```python
from build123d import *

# Parameters (mm, degrees)
SKETCH008_W     = 36.83
SKETCH008_H     = 68.58
PAD006_DEPTH    = 8.89
SKETCH009_W     = 31.75
SKETCH009_H     = 62.23
POCKET001_DEPTH = 6.35
SKETCH010_R     = 5.715
SKETCH010_W     = 6.35
SKETCH010_H     = 2.54
SKETCH010_W_2   = 5.08
SKETCH010_W_3   = 2.54
SKETCH010_H_2   = 6.35
SKETCH010_H_3   = 3.81
PAD007_DEPTH    = 6.35
POCKET002_DEPTH = 1.5875
SKETCH012_W     = 36.83
SKETCH012_H     = 68.58
SKETCH012_W_2   = 31.75
SKETCH012_H_2   = 62.23
SKETCH012_R     = 5.715
PAD008_DEPTH    = 3.81
SKETCH013_R     = 5.08
POCKET003_DEPTH = 5.08
SKETCH014_R     = 1.651
POCKET004_DEPTH = 12.701
SKETCH015_R     = 3.175
POCKET005_DEPTH = 10.16
SKETCH016_R     = 3.175
POCKET006_DEPTH = 4.7625
SKETCH017_W     = 5.715
SKETCH017_H     = 1.143
PAD009_DEPTH    = 1.27
POCKET007_DEPTH = 10.16
SKETCH019_W     = 29.21
SKETCH019_H     = 1.143
SKETCH019_W_2   = 5.08
PAD010_DEPTH    = 1.27
FILLET004_R     = 1.27
FILLET005_R     = 0.762


with BuildPart() as part:
    # Sketch008 → Pad006 (new body)
    with BuildSketch(Plane.XY):
        with Locations((15.875, 31.75)):
            Rectangle(SKETCH008_W, SKETCH008_H)
    extrude(amount=-PAD006_DEPTH)

    # Sketch009 (on Face5 of Pad006) → Pocket001 (cut)
    with BuildSketch(Plane.XY):
        with Locations((15.875, 31.115)):
            Rectangle(SKETCH009_W, SKETCH009_H)
    extrude(amount=-POCKET001_DEPTH, mode=Mode.SUBTRACT)

    # Sketch010 (on Face11 of Pocket001) → Pad007 (join)
    with BuildSketch(Plane.XY.offset(-6.35)):
        with Locations((7.62, 22.225)):
            Circle(SKETCH010_R)
        with Locations((7.62, 50.8)):
            Circle(SKETCH010_R)
        with Locations((24.13, 50.8)):
            Circle(SKETCH010_R)
        with Locations((3.175, 33.02)):
            Rectangle(SKETCH010_W, SKETCH010_H)
        with Locations((29.21, 33.02)):
            Rectangle(SKETCH010_W_2, SKETCH010_H)
        with Locations((3.175, 9.525)):
            Rectangle(SKETCH010_W, SKETCH010_H)
        with Locations((29.21, 9.525)):
            Rectangle(SKETCH010_W_2, SKETCH010_H)
        with Locations((15.875, 37.465)):
            Rectangle(SKETCH010_W_3, SKETCH010_H_2)
        with Locations((13.97, 1.905)):
            Rectangle(SKETCH010_W_3, SKETCH010_H_3)
    extrude(amount=PAD007_DEPTH)

    # Sketch011 (on Face4 of Pad007) → Pocket002 (cut)
    with BuildSketch(Plane.XY):
        with BuildLine():
            Line((2.286, 0), (31.369, 0))
            Line((31.369, 0), (31.369, 38.608))
            Line((31.369, 38.608), (2.286, 38.608))
            Line((2.286, 38.608), (2.286, 25.670424))
            ThreePointArc((2.286, 25.670424), (1.27, 22.225), (2.286, 18.779576))
            Line((2.286, 0), (2.286, 18.779576))
        make_face()
    extrude(amount=-POCKET002_DEPTH, mode=Mode.SUBTRACT)

    # Sketch012 (on Face4 of Pocket002) → Pad008 (join)
    with BuildSketch(Plane.XY):
        with Locations((15.875, 31.75)):
            Rectangle(SKETCH012_W, SKETCH012_H)
        with Locations((15.875, 31.115)):
            Rectangle(SKETCH012_W_2, SKETCH012_H_2, mode=Mode.SUBTRACT)
        with Locations((7.62, 50.8)):
            Circle(SKETCH012_R)
        with Locations((24.13, 50.8)):
            Circle(SKETCH012_R)
    extrude(amount=PAD008_DEPTH)

    # Sketch013 (on Face4 of Pad008) → Pocket003 (cut)
    with BuildSketch(Plane.XZ.offset(2.54)):
        with Locations((23.495, 3.81)):
            Circle(SKETCH013_R)
        with BuildLine():
            Line((2.54, 3.81), (3.556, 2.54))
            Line((3.556, 2.54), (4.826, 2.54))
            ThreePointArc((4.826, 2.54), (7.62, -0.254), (10.414, 2.54))
            Line((10.414, 2.54), (11.684, 2.54))
            Line((11.684, 2.54), (12.7, 3.81))
            Line((12.7, 3.81), (2.54, 3.81))
        make_face()
    extrude(amount=-POCKET003_DEPTH, mode=Mode.SUBTRACT)

    # Sketch014 (on Face11 of Pocket003) → Pocket004 (cut, through all)
    with BuildSketch(Plane.XY.offset(3.81)):
        with Locations((7.62, 50.8)):
            Circle(SKETCH014_R)
        with Locations((24.13, 50.8)):
            Circle(SKETCH014_R)
        with Locations((7.62, 22.225)):
            Circle(SKETCH014_R)
    extrude(amount=-POCKET004_DEPTH, mode=Mode.SUBTRACT)

    # Sketch015 (on Face8 of Pocket004) → Pocket005 (cut)
    with BuildSketch(Plane(origin=(0, 0, -8.89), x_dir=(1, 0, 0), z_dir=(0, 0, -1))):
        with Locations((7.62, -50.8)):
            Circle(SKETCH015_R)
        with Locations((24.13, -50.8)):
            Circle(SKETCH015_R)
    extrude(amount=-POCKET005_DEPTH, mode=Mode.SUBTRACT)

    # Sketch016 (on Face8 of Pocket005) → Pocket006 (cut)
    with BuildSketch(Plane(origin=(0, 0, -8.89), x_dir=(1, 0, 0), z_dir=(0, 0, -1))):
        with Locations((7.62, -22.225)):
            Circle(SKETCH016_R)
    extrude(amount=-POCKET006_DEPTH, mode=Mode.SUBTRACT)

    # Sketch017 (on Face11 of Pocket006) → Pad009 (join)
    with BuildSketch(Plane.XY.offset(3.81)):
        Polygon((0, 62.23), (-1.143, 62.23), (-1.143, -1.143), (2.54, -1.143), (2.54, 0), (0, 0), align=None)
        Polygon((31.75, 62.23), (31.75, 0), (28.575, 0), (28.575, -1.143), (32.893, -1.143), (32.893, 62.23), align=None)
        with Locations((15.5575, -0.5715)):
            Rectangle(SKETCH017_W, SKETCH017_H)
    extrude(amount=PAD009_DEPTH)

    # Sketch018 (on Face11 of Pad009) → Pocket007 (cut)
    with BuildSketch(Plane.XY.offset(3.81)):
        Polygon((1.27, 66.04), (1.27, 64.897), (0, 64.897), (0, 63.373), (1.27, 63.373), (1.27, 62.23), (30.48, 62.23), (30.48, 63.373), (31.75, 63.373), (31.75, 64.897), (30.48, 64.897), (30.48, 66.04), align=None)
    extrude(amount=-POCKET007_DEPTH, mode=Mode.SUBTRACT)

    # Sketch019 (on Face63 of Pocket007) → Pad010 (join)
    with BuildSketch(Plane.XY.offset(-6.35)):
        with Locations((15.875, 65.4685)):
            Rectangle(SKETCH019_W, SKETCH019_H)
        with Locations((3.81, 62.8015)):
            Rectangle(SKETCH019_W_2, SKETCH019_H)
        with Locations((27.94, 62.8015)):
            Rectangle(SKETCH019_W_2, SKETCH019_H)
    extrude(amount=PAD010_DEPTH)

    # Fillet004
    fillet004_edges = [part.edges().sort_by_distance(p)[0] for p in [
        (-2.54, -2.54, 1.905),
        (-2.54, -2.54, -4.445),
        (34.29, -2.54, -4.445),
        (34.29, -2.54, 1.905),
        (34.29, 66.04, 1.905),
        (34.29, 66.04, -4.445),
        (15.875, -2.54, -8.89),
        (34.29, 31.75, -8.89),
        (-2.54, 31.75, -8.89),
        (15.875, 66.04, -8.89),
        (-2.54, 66.04, 1.905),
        (-2.54, 66.04, -4.445),
    ]]
    fillet(fillet004_edges, radius=FILLET004_R)

    # Fillet005
    fillet005_edges = [part.edges().sort_by_distance(p)[0] for p in [
        (4.445, 22.225, -8.89),
        (20.955, 50.8, -8.89),
        (4.445, 50.8, -8.89),
    ]]
    fillet(fillet005_edges, radius=FILLET005_R)


solid = part.part
```
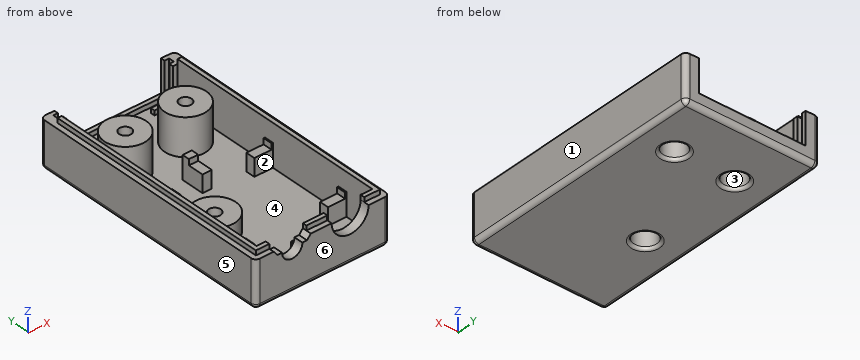
Geometry: final body of the model. Coordinates: model frame, mm. Face numbers are marked on the shaded views. A direction names the side the tool comes from. Round coordinates to 2 decimals unless told otherwise and drop trailing zeros. Write each loop counter-clockwise with the first axis right and the second up, starting at its lowest first coordinate (ties: lowest second). Pieces come first, ordered by that corner, then holes.
Item 1: Section query A-A (x = 7.62). Give the number of separate pieces and of enclosed holes in the cut face, plus the area to 3 significant figures.
Item 2: Mould query, pull axis Y, two halves, no side actions, for the marked faces 4, 5 and 6. Classes: +Y half, -Y half, draft (parallel to the pull), parting line (faces both ways), or undercut.
Item 3: Pin query (flat end, axial travel): P1, Ø9, axis at x = 10.5, y = 19.5, coming from the +Z side; P2, Ø1.9, axis at x = 4.5, z = -2, coming from the +Y side; P3, Ø1.1, axis at x = 1, y = 9.5, coming from the +Z side. Return the tip coordinate at first contact, or that it passes through.
Item 4: Section query C-C (x = 24.13). Return loops of the section in (y, z) (3 decimals).
Item 5: Section query B-B (y = 15). Return loops of the section in (x, z), plus the area to 3 significant figures.
Item 6: Set-up query: the marked faces 1, 2 and 3. Return all of +Z, -Z, +X, -X, +Y, -Y with unobstructed straight access to the full face (end or side cutting, diameter ignored); none if empty.
Item 7: Material intervals for L1, parallel to X at y = 37, z = -5.75 (3 decimals); L2, parallel to Y at x = 7.62, z = -6.05 (3 decimals); L3, parallel to Y at x = 31, z = -2.75 (3 decimals), sorted ascending.
Completed:
1. separate pieces: 3
1. enclosed holes: 0
1. area: 249 mm2
2. face 4: undercut
2. face 5: draft
2. face 6: -Y half
3. P1: stops at z = -1.59
3. P2: stops at y = 56.09
3. P3: stops at z = 0
4. outline: (-2.54, -7.62) arc R1.27 ccw to (-1.27, -8.89) - (46.863, -8.89) arc R0.762 ccw to (47.625, -8.128) - (47.625, 1.27) - (49.149, 1.27) - (49.149, 3.81) - (45.085, 3.81) - (45.085, -6.35) - (0, -6.35) - (0, -1.23) - (-2.54, -1.23) - close; (52.451, 1.27) - (53.975, 1.27) - (53.975, -8.128) arc R0.762 ccw to (54.737, -8.89) - (64.77, -8.89) arc R1.27 ccw to (66.04, -7.62) - (66.04, -5.08) - (64.897, -5.08) - (64.897, -6.35) - (56.515, -6.35) - (56.515, 3.81) - (52.451, 3.81) - close
5. outline: (-2.54, -7.62) arc R1.27 ccw to (-1.27, -8.89) - (33.02, -8.89) arc R1.27 ccw to (34.29, -7.62) - (34.29, 3.81) - (32.89, 3.81) - (32.89, 5.08) - (31.75, 5.08) - (31.75, -6.35) - (0, -6.35) - (0, 5.08) - (-1.14, 5.08) - (-1.14, 3.81) - (-2.54, 3.81) - close
5. area: 147 mm2
6. face 1: +Z, -Z, +X, +Y, -Y
6. face 2: +Z
6. face 3: -Z
7. L1: x = -2.54 to 0, 14.605 to 17.145, 31.75 to 34.29
7. L2: y = -2.54 to 0, 16.51 to 19.05, 25.4 to 27.94, 45.085 to 47.625, 53.975 to 56.515, 64.897 to 66.04
7. L3: y = -2.54 to 0, 8.255 to 10.795, 31.75 to 34.29, 62.23 to 63.373, 64.897 to 66.04
